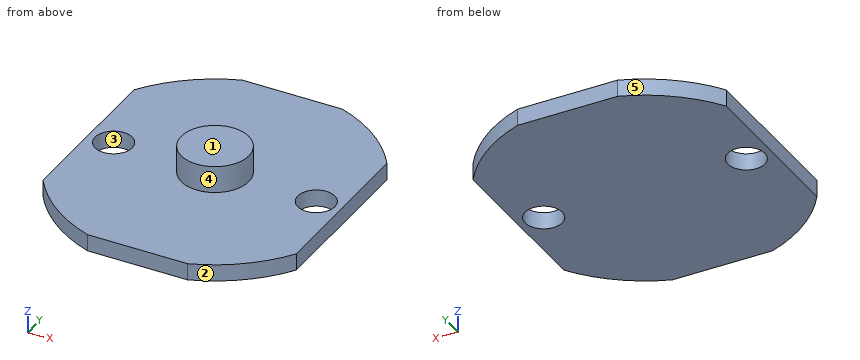
```python
from build123d import *

# Parameters (mm, degrees)
SKETCH_1_R          = 9
SKETCH_1_R_2        = 1.1
EXTRUDE_1_DEPTH     = 1
SKETCH_2_W          = 32.389432278
SKETCH_2_H          = 26.120675296
SKETCH_2_W_2        = 15
SKETCH_2_H_2        = 17
CUT_EXTRUDE_1_DEPTH = 2
SKETCH_3_R          = 2
EXTRUDE_2_DEPTH     = 1.6


with BuildPart() as part:
    # 草图1 → 凸台-拉伸1 (new body)
    with BuildSketch(Plane.XY):
        Circle(SKETCH_1_R)
        with Locations((6, 0)):
            Circle(SKETCH_1_R_2, mode=Mode.SUBTRACT)
        with Locations((-6, 0)):
            Circle(SKETCH_1_R_2, mode=Mode.SUBTRACT)
    extrude(amount=EXTRUDE_1_DEPTH)

    # 草图2 → 切除-拉伸1 (cut)
    with BuildSketch(Plane.XY.offset(1)):
        Rectangle(SKETCH_2_W, SKETCH_2_H)
        Rectangle(SKETCH_2_W_2, SKETCH_2_H_2, mode=Mode.SUBTRACT)
    extrude(amount=-CUT_EXTRUDE_1_DEPTH, mode=Mode.SUBTRACT)

    # 草图3 → 凸台-拉伸2 (add)
    with BuildSketch(Plane.XY.offset(1)):
        Circle(SKETCH_3_R)
    extrude(amount=EXTRUDE_2_DEPTH)


solid = part.part
```
Design review of the part built by this model. Coordinates are the model's own, in mm. Face numbers are marked on the shaded views. A direction names the side the tool comes from. Give positions to 0.01 mm unless a question says otherwise; leave off trailing zeros. Write each loop counter-clockwise with the first axis right and the second up, starting at its lowest first coordinate (ties: lowest second). Pieces come first, ordered by that corner, then holes. Notation, with made-up numbers: (60, 43) -> (102, 43) arc R22 cw to (102, 68) -> close; hole circle Ø8 at (64.25, 72). An arc over 180 degrees is marked (long way). Answer in a Markdown table with one row per item.
(1) Consider section B-B (x = 0). State the section outline as (y, z) points.
Results:
| item | result |
|---|---|
| outline | (-8.5, 0) -> (8.5, 0) -> (8.5, 1) -> (2, 1) -> (2, 2.6) -> (-2, 2.6) -> (-2, 1) -> (-8.5, 1) -> close |
(2) For the marked faces 4 and 5, list the 3-axis set-ups (+Z, -Z, +X, -X, +Y, -Y) from which the entire face can be reached by the end or side of a thin tool; tool diameter is ignored.
Results:
| item | result |
|---|---|
| face 4 | +Z |
| face 5 | +Z, -Z, -X, +Y |
(3) Consider section C-C (x = -6). State the section outline as (y, z) points.
Results:
| item | result |
|---|---|
| outline | (-6.71, 0) -> (-1.1, 0) -> (-1.1, 1) -> (-6.71, 1) -> close; (1.1, 0) -> (6.71, 0) -> (6.71, 1) -> (1.1, 1) -> close |
(4) Consider section A-A (y = 0). State the section outline as (x, z) points, then the cut area to 3 significant figures.
Results:
| item | result |
|---|---|
| outline | (-7.5, 0) -> (-7.1, 0) -> (-7.1, 1) -> (-7.5, 1) -> close; (-4.9, 0) -> (4.9, 0) -> (4.9, 1) -> (2, 1) -> (2, 2.6) -> (-2, 2.6) -> (-2, 1) -> (-4.9, 1) -> close; (7.1, 0) -> (7.5, 0) -> (7.5, 1) -> (7.1, 1) -> close |
| area | 17.0 mm2 |
(5) Clearance check with a flat-ended pin moving along its axis: pin 1 (3.5 mm diameter, centred on x = 6, y = 0, fed in from +Z). State where the tip first meets the part, or that it passes through.
Results:
| item | result |
|---|---|
| pin 1 | z = 1 |
(6) Consider section D-D (z = 1.9). State the section outline as (x, y) points.
Results:
| item | result |
|---|---|
| outline | circle Ø4 at (0, 0) |
(7) To check wall thickness, follow probe 1 along X at (y, z) = (-0.5, 0.3); probe 2 along Z at (x, y) = (-3.75, 7.5); probe 3 along Y at (x, z) = (-6, 0.8). State the ranges of each line that lie inside material, in increasing order.
Results:
| item | result |
|---|---|
| probe 1 | -7.5 to -6.98, -5.02 to 5.02, 6.98 to 7.5 |
| probe 2 | 0 to 1 |
| probe 3 | -6.71 to -1.1, 1.1 to 6.71 |
(8) Mouldability with a two-part tool opening along Y and no side actions: class the marked faces 1, 2 and 3 as +Y half, -Y half, draft (parallel to the pull), parting line (faces both ways), or undercut.
Results:
| item | result |
|---|---|
| face 1 | draft |
| face 2 | -Y half |
| face 3 | undercut |
